```python
from build123d import *

# Parameters (mm, degrees)
BOSS_EXTRUDE1_DEPTH     = 12.5
SKETCH2_W               = 10.5
SKETCH2_H               = 41.75
BOSS_EXTRUDE2_DEPTH     = 5
CUT_EXTRUDE1_DEPTH      = 25
CUT_EXTRUDE1_DEPTH_BACK = 6
CUT_EXTRUDE2_START      = 4
CUT_EXTRUDE2_DEPTH      = 3


with BuildPart() as part:
    # Sketch1 → Boss-Extrude1 (new body, symmetric)
    with BuildSketch(Plane(origin=(0, 0, 0), x_dir=(0, 0, -1), z_dir=(1, 0, 0))):
        with BuildLine():
            Line((0, 0), (70, 0))
            Line((70, 0), (70, 14))
            ThreePointArc((70, 14), (60, 24), (50, 14))
            Line((50, 14), (50, 4))
            Line((50, 4), (20, 4))
            Line((20, 4), (20, 14))
            ThreePointArc((20, 14), (10, 24), (0, 14))
            Line((0, 14), (0, 0))
        make_face()
    extrude(amount=BOSS_EXTRUDE1_DEPTH, both=True)

    # Sketch2 → Boss-Extrude2 (add)
    with BuildSketch(Plane(origin=(0, 0, 0), x_dir=(1, 0, 0), z_dir=(0, 1, 0))):
        with BuildLine():
            ThreePointArc((-5.25, 41.75), (0, 47), (5.25, 41.75))
            Line((5.25, 41.75), (-5.25, 41.75))
        make_face()
        with Locations((0, 20.875)):
            Rectangle(SKETCH2_W, SKETCH2_H)
    extrude(amount=-BOSS_EXTRUDE2_DEPTH)

    # Sketch4 → Cut-Extrude1 (cut, two sides)
    with BuildSketch(Plane(origin=(0, 0, 0), x_dir=(1, 0, 0), z_dir=(0, 1, 0))) as cut_extrude1_sk:
        with BuildLine():
            Line((1.625, 31), (1.625, 25))
            ThreePointArc((1.625, 25), (0, 23.375), (-1.625, 25))
            Line((-1.625, 25), (-1.625, 31))
            ThreePointArc((-1.625, 31), (0, 32.625), (1.625, 31))
        make_face()
        with BuildLine():
            Line((1.625, 46), (1.625, 40))
            ThreePointArc((1.625, 40), (0, 38.375), (-1.625, 40))
            Line((-1.625, 40), (-1.625, 46))
            ThreePointArc((-1.625, 46), (0, 47.625), (1.625, 46))
        make_face()
    extrude(amount=CUT_EXTRUDE1_DEPTH, mode=Mode.SUBTRACT)
    extrude(cut_extrude1_sk.sketch, amount=-CUT_EXTRUDE1_DEPTH_BACK, mode=Mode.SUBTRACT)

    # Sketch4<3> → Cut-Extrude2 (cut)
    with BuildSketch(Plane(origin=(0, 0, 0), x_dir=(1, 0, 0), z_dir=(0, 1, 0)).offset(CUT_EXTRUDE2_START)):
        with BuildLine():
            Line((-2.5, 31), (-2.5, 25))
            ThreePointArc((-2.5, 25), (0, 22.5), (2.5, 25))
            Line((2.5, 25), (2.5, 31))
            ThreePointArc((2.5, 31), (0, 33.5), (-2.5, 31))
        make_face()
        with BuildLine():
            ThreePointArc((1.625, 31), (0, 32.625), (-1.625, 31))
            Line((-1.625, 31), (-1.625, 25))
            ThreePointArc((-1.625, 25), (0, 23.375), (1.625, 25))
            Line((1.625, 25), (1.625, 31))
        make_face(mode=Mode.SUBTRACT)
        with BuildLine():
            Line((-2.5, 46), (-2.5, 40))
            ThreePointArc((-2.5, 40), (0, 37.5), (2.5, 40))
            Line((2.5, 40), (2.5, 46))
            ThreePointArc((2.5, 46), (0, 48.5), (-2.5, 46))
        make_face()
        with BuildLine():
            ThreePointArc((1.625, 46), (0, 47.625), (-1.625, 46))
            Line((-1.625, 46), (-1.625, 40))
            ThreePointArc((-1.625, 40), (0, 38.375), (1.625, 40))
            Line((1.625, 40), (1.625, 46))
        make_face(mode=Mode.SUBTRACT)
    extrude(amount=-CUT_EXTRUDE2_DEPTH, mode=Mode.SUBTRACT)


solid = part.part
```
Source: CAD feature listing. Evaluate the final solid. Frame: model axes, mm. A direction names the side the tool comes from. Round coordinates to 2 decimals unless told otherwise and drop trailing zeros. Loops run counter-clockwise (first coordinate to the right, second up) from the corner with the lowest first, then second, coordinate; pieces in that order, holes last.
(1) Section query C-C (x = 0). Output: boundary loops of the cut face in (y, z) (3 decimals).
From the geometry:
outline: (-5, -38.375) - (1, -38.375) - (1, -37.5) - (4, -37.5) - (4, -33.5) - (1, -33.5) - (1, -32.625) - (-5, -32.625) - close; (-5, -23.375) - (1, -23.375) - (1, -22.5) - (4, -22.5) - (4, -20) - (14, -20) arc R10 ccw to (14, 0) - (-5, 0) - close; (0, -70) - (14, -70) arc R10 ccw to (14, -50) - (4, -50) - (4, -48.5) - (1, -48.5) - (1, -47.625) - (0, -47.625) - close
(2) Access query for faces 1 (the flat face through (-2.5, 3, -43)), 2 (the flat face through (1.625, -2, -43)), 3 (the cylindrical face through (-4.2, -2.5, -44.9)). Directions: +Z, -Z, +X, -X, +Y, -Y. A direction counts if a zero-diameter tool reaches every point of the face in a straight line with its end or side. Return the directions, or none.
From the geometry:
face 1: +Y
face 2: +Y, -Y
face 3: -Z, -X, -Y
(3) Section query A-A (y = 2.75). Output: boundary loops of the cut face in (x, z).
From the geometry:
outline: (-12.5, -70) - (12.5, -70) - (12.5, 0) - (-12.5, 0) - close; hole (-2.5, -46) arc R2.5 ccw to (2.5, -46) - (2.5, -40) arc R2.5 ccw to (-2.5, -40) - close; hole (-2.5, -31) arc R2.5 ccw to (2.5, -31) - (2.5, -25) arc R2.5 ccw to (-2.5, -25) - close
(4) Pull-direction query (X, two-part tool) for faces 4 (the flat face through (0, 7, 0)), 5 (the cylindrical face through (4.152, -2.465, -44.963)), 6 (the cylindrical face through (0.036, -1.958, -23.375)); classes: +X half, -X half, draft (parallel to the pull), parting line (faces both ways), or undercut.
From the geometry:
face 4: draft
face 5: +X half
face 6: undercut
(5) Material intervals for probe 1 along Z at (x, y) = (-5.25, 5); probe 2 along X at (y, z) = (-3.25, -29.5) (3 decimals); probe 3 along Y at (x, z) = (11.5, -37.5), sorted ascending.
From the geometry:
probe 1: z = -70 to -50, -20 to 0
probe 2: x = -5.25 to -1.625, 1.625 to 5.25
probe 3: y = 0 to 4
(6) Section query D-D (y = 13). Output: boundary loops of the cut face in (x, z).
From the geometry:
outline: (-12.5, -70) - (12.5, -70) - (12.5, -50) - (-12.5, -50) - close; (-12.5, -20) - (12.5, -20) - (12.5, 0) - (-12.5, 0) - close
(7) Section query B-B (z = -27.5). Output: boundary loops of the cut face in (x, y) (3 decimals).
From the geometry:
outline: (-12.5, 0) - (-5.25, 0) - (-5.25, -5) - (-1.625, -5) - (-1.625, 1) - (-2.5, 1) - (-2.5, 4) - (-12.5, 4) - close; (1.625, -5) - (5.25, -5) - (5.25, 0) - (12.5, 0) - (12.5, 4) - (2.5, 4) - (2.5, 1) - (1.625, 1) - close
(8) Contact query for flat-ended pins moving along their axis: pin 1 Ø6 at (x, z) = (2.5, -29.5) entering from +Y; pin 2 Ø1.8 at (y, z) = (-2, -27) entering from +X; pin 3 Ø6 at (x, z) = (-9, -59) entering from -Y. Output: stop coordinate, or through.
From the geometry:
pin 1: stops at y = 4
pin 2: stops at x = 5.25
pin 3: stops at y = 0
